```python
from build123d import *

# Parameters (mm, degrees)
SKETCH1_W           = 100.1
SKETCH1_H           = 120
SKETCH1_R           = 2.75
SKETCH1_R_2         = 2.11
SKETCH1_W_2         = 22.25
SKETCH1_H_2         = 10.95
BOSS_EXTRUDE1_DEPTH = 2
SKETCH2_W           = 2
SKETCH2_H           = 115.8
BOSS_EXTRUDE2_DEPTH = 16
SKETCH4_W           = 95.1
SKETCH4_H           = 2
BOSS_EXTRUDE3_DEPTH = 16
SKETCH5_W           = 2.5
SKETCH5_H           = 2.1
CUT_EXTRUDE1_DEPTH  = 2
SKETCH6_W           = 7
SKETCH6_H           = 28.4
CUT_EXTRUDE2_DEPTH  = 3
FILLET2_R           = 2


with BuildPart() as part:
    # Sketch1 → Boss-Extrude1 (new body)
    with BuildSketch(Plane.XY):
        with Locations((50.05, -60)):
            Rectangle(SKETCH1_W, SKETCH1_H)
        with Locations((10, -10)):
            Circle(SKETCH1_R, mode=Mode.SUBTRACT)
        with Locations((90.1, -10)):
            Circle(SKETCH1_R, mode=Mode.SUBTRACT)
        with Locations((10, -110)):
            Circle(SKETCH1_R, mode=Mode.SUBTRACT)
        with Locations((6.05, -18.5)):
            Circle(SKETCH1_R_2, mode=Mode.SUBTRACT)
        with Locations((6.05, -83.5)):
            Circle(SKETCH1_R_2, mode=Mode.SUBTRACT)
        with Locations((94.05, -18.5)):
            Circle(SKETCH1_R_2, mode=Mode.SUBTRACT)
        with Locations((94.05, -83.5)):
            Circle(SKETCH1_R_2, mode=Mode.SUBTRACT)
        with Locations((20.05, -10)):
            Circle(SKETCH1_R_2, mode=Mode.SUBTRACT)
        with Locations((80.05, -10)):
            Circle(SKETCH1_R_2, mode=Mode.SUBTRACT)
        with Locations((20.05, -110)):
            Circle(SKETCH1_R_2, mode=Mode.SUBTRACT)
        with Locations((80.05, -110)):
            Circle(SKETCH1_R_2, mode=Mode.SUBTRACT)
        with Locations((90.1, -110)):
            Circle(SKETCH1_R, mode=Mode.SUBTRACT)
        with Locations((50.05, -10)):
            Circle(SKETCH1_R, mode=Mode.SUBTRACT)
        with Locations((35.275, -26.925)):
            Rectangle(SKETCH1_W_2, SKETCH1_H_2, mode=Mode.SUBTRACT)
        with Locations((65.725, -26.925)):
            Rectangle(SKETCH1_W_2, SKETCH1_H_2, mode=Mode.SUBTRACT)
    extrude(amount=BOSS_EXTRUDE1_DEPTH)

    # Sketch2 → Boss-Extrude2 (add)
    with BuildSketch(Plane.XY.offset(2)):
        with Locations((1, -60)):
            Rectangle(SKETCH2_W, SKETCH2_H)
    boss_extrude2 = extrude(amount=BOSS_EXTRUDE2_DEPTH)

    # Mirror1: Boss-Extrude2 across plane
    add(boss_extrude2.mirror(Plane(origin=(50.05, 0, 0), x_dir=(0, 0, 1), z_dir=(1, 0, 0))))

    # Sketch4 → Boss-Extrude3 (add)
    with BuildSketch(Plane.XY.offset(2)):
        with Locations((50.05, -1)):
            Rectangle(SKETCH4_W, SKETCH4_H)
        with Locations((50.05, -119)):
            Rectangle(SKETCH4_W, SKETCH4_H)
    extrude(amount=BOSS_EXTRUDE3_DEPTH)

    # Sketch5 → Cut-Extrude1 (cut)
    with BuildSketch(Plane(origin=(0, 0, 0), x_dir=(-1, 0, 0), z_dir=(0, 0, -1))):
        with Locations((-1.25, -1.05)):
            Rectangle(SKETCH5_W, SKETCH5_H)
        with Locations((-98.85, -118.95)):
            Rectangle(SKETCH5_W, SKETCH5_H)
        with Locations((-1.25, -118.95)):
            Rectangle(SKETCH5_W, SKETCH5_H)
        with Locations((-98.85, -1.05)):
            Rectangle(SKETCH5_W, SKETCH5_H)
    extrude(amount=-CUT_EXTRUDE1_DEPTH, mode=Mode.SUBTRACT)

    # Sketch6 → Cut-Extrude2 (cut)
    with BuildSketch(Plane.ZY):
        with Locations((3.5, -51.4)):
            Rectangle(SKETCH6_W, SKETCH6_H)
    extrude(amount=-CUT_EXTRUDE2_DEPTH, mode=Mode.SUBTRACT)

    # Fillet2
    fillet2_edges = [part.edges().sort_by_distance(p)[0] for p in [
        (0, -19.65, 0),
        (100.1, -60, 0),
        (50.05, -120, 0),
        (50.05, 0, 0),
        (0, -91.75, 0),
    ]]
    fillet(fillet2_edges, radius=FILLET2_R)


solid = part.part
```
Geometry check sheet. Reference: the model listing, model coordinates, mm. A direction names the side the tool comes from. Give positions to 0.01 mm unless a question says otherwise; leave off trailing zeros. Write each loop counter-clockwise with the first axis right and the second up, starting at its lowest first coordinate (ties: lowest second). Pieces come first, ordered by that corner, then holes. Notation, with made-up numbers: (-11.75, -4.5) - (-2.75, -4.5) arc R12 ccw to (-2.75, 14.5) - close; hole circle Ø11 at (12.25, 27). An arc over 180 degrees is marked (long way). Use a Markdown table: item, result.
Q1. Draft check along Y on faces 1 (the face through (1, -117.9, 9)), 2 (the face through (1, -37.2, 3)), 3 (the face through (49, -59, 0)). Enter one of: pulls with the +Y half, pulls with the -Y half, needs draft (parallel to the pull), parting line crosses it, or undercut.
Computed:
| item | result |
|---|---|
| face 1 | pulls with the -Y half |
| face 2 | undercut |
| face 3 | needs draft |
Q2. Set-up check for faces 4 (the face through (2, -61, 10)), 5 (the face through (49, -2, 10)), 6 (the face through (49, -59, 2)), 7 (the face through (92.72, -9.17, 0.99)), 8 (the face through (99, -2.1, 9)): record each of +Z, -Z, +X, -X, +Y, -Y from which the full face is reachable in a straight line by a thin tool's end or side.
Computed:
| item | result |
|---|---|
| face 4 | +Z, +Y, -Y |
| face 5 | +Z, +X, -X |
| face 6 | +Z |
| face 7 | +Z, -Z |
| face 8 | +Z, -Z, +X, +Y |
Q3. Go/stop test with flat-tipped pins: P1, Ø2, axis at x = 99, z = 6.5, coming from the -Y side; P2, Ø5, axis at x = 20.05, y = -110, coming from the +Z side; P3, Ø5, axis at y = -60.5, z = 2, coming from the -X side; P4, Ø3, axis at x = 2, z = 8.5, coming from the +Y side. Record where each tip stops, or that it passes through.
Computed:
| item | result |
|---|---|
| P1 | stops at y = -117.9 |
| P2 | stops at z = 2 |
| P3 | stops at x = 3 |
| P4 | stops at y = 0 |
Q4. Section check C-C, the plane x = 28. Enter the section's corners in (y, z), then the cut area to 3 significant figures.
Computed:
| item | result |
|---|---|
| outline | (-120, 2) arc R2 ccw to (-118, 0) - (-32.4, 0) - (-32.4, 2) - (-118, 2) - (-118, 18) - (-120, 18) - close; (-21.45, 0) - (-2, 0) arc R2 ccw to (0, 2) - (0, 18) - (-2, 18) - (-2, 2) - (-21.45, 2) - close |
| area | 280 mm² |
Q5. Section check A-A, the plane y = -26.5. Enter the section's corners in (x, z).
Computed:
| item | result |
|---|---|
| outline | (0, 2) arc R2 ccw to (2, 0) - (24.15, 0) - (24.15, 2) - (2, 2) - (2, 18) - (0, 18) - close; (46.4, 0) - (54.6, 0) - (54.6, 2) - (46.4, 2) - close; (76.85, 0) - (98.1, 0) arc R2 ccw to (100.1, 2) - (100.1, 18) - (98.1, 18) - (98.1, 2) - (76.85, 2) - close |
Q6. Thickness scan on L1, parallel to X at y = -98.5, z = 16.5; L2, parallel to Y at x = 10, z = 1.5; L3, parallel to Y at x = 90.1, z = 0.8. Record the ranges inside material, lowest first. Write a range as [from, to].
Computed:
| item | result |
|---|---|
| L1 | x = [0, 2], [98.1, 100.1] |
| L2 | y = [-119.94, -112.75], [-107.25, -12.75], [-7.25, -0.06] |
| L3 | y = [-119.6, -112.75], [-107.25, -12.75], [-7.25, -0.4] |
Q7. Section check D-D, the plane z = 15. Enter the section's corners in (x, y), then the cut area to 3 significant figures.
Computed:
| item | result |
|---|---|
| outline | (0, -117.9) - (2, -117.9) - (2, -2.1) - (0, -2.1) - close; (2.5, -120) - (97.6, -120) - (97.6, -118) - (2.5, -118) - close; (2.5, -2) - (97.6, -2) - (97.6, 0) - (2.5, 0) - close; (98.1, -117.9) - (100.1, -117.9) - (100.1, -2.1) - (98.1, -2.1) - close |
| area | 844 mm² |
Q8. Section check B-B, the plane x = 80.05. Enter the section's corners in (y, z), then the cut area to 3 significant figures.
Computed:
| item | result |
|---|---|
| outline | (-120, 2) arc R2 ccw to (-118, 0) - (-112.11, 0) - (-112.11, 2) - (-118, 2) - (-118, 18) - (-120, 18) - close; (-107.89, 0) - (-12.11, 0) - (-12.11, 2) - (-107.89, 2) - close; (-7.89, 0) - (-2, 0) arc R2 ccw to (0, 2) - (0, 18) - (-2, 18) - (-2, 2) - (-7.89, 2) - close |
| area | 285 mm² |
